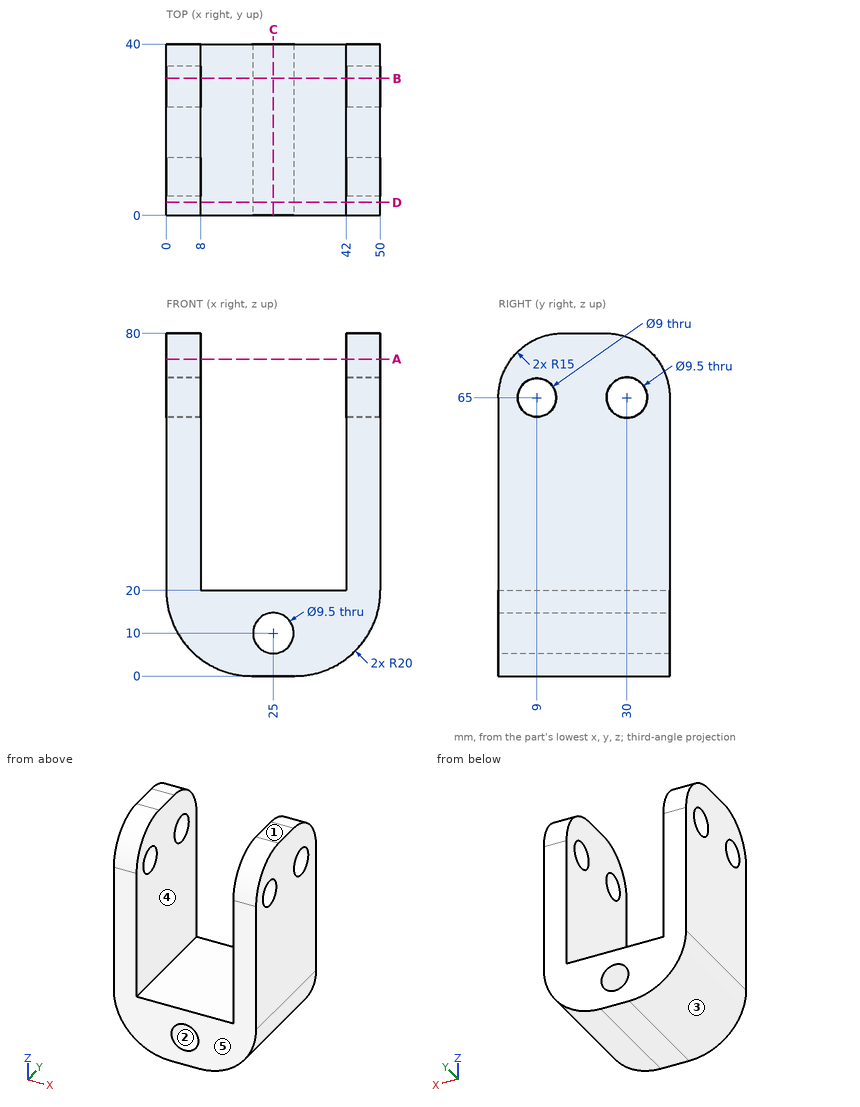
Geometry: see drawing. Coordinates: mm, zero at the bounding-box minimum. A direction names the side the tool comes from. Round coordinates to 2 decimals unless told otherwise and drop trailing zeros. Loops run counter-clockwise (first coordinate to the right, second up) from the corner with the lowest first, then second, coordinate; pieces in that order, holes last. Notation, with made-up numbers: M 4.5,52.25 L 54.5,52.25 A28 cw 54.5,85.25 Z; hole C 45,-9 d4. An arc over 180 degrees is marked long. Use a Markdown table: item, result. Add a question column.
1. Contact query for flat-ended pins moving along their axis: P1, Ø8.5, axis at y = 30, z = 65, coming from the -X side; P2, Ø10, axis at x = 24, y = 31, coming from the +Z side; P3, Ø10, axis at x = 44, y = 35, coming from the +Z side; P4, Ø10, axis at x = 11, y = 4.5, coming from the -Z side. Output: stop coordinate, or through.
2. Section query D-D on y = 3. Return the cut outline in (x, z), then the cut area to 3 significant figures.
3. Section query B-B on y = 32. Return the cut outline in (x, z).
4. Section query A-A on z = 74. Return the cut outline in (x, y).
5. Line query: line 1 (Y direction, x = 3.75, z = 65); line 2 (X direction, y = 25, z = 45); line 3 (Z direction, x = 42.5, y = 32). Output: solid intervals per line, ascending.
6. Reachability of the marked faces 4 and 5 from +Z, -Z, +X, -X, +Y, -Y: full face, straight path, thin tool, end or side. Return the list, or none.
7. Mould query, pull axis X, two halves, no side actions, for the marked faces 1, 2 and 3. Classes: pulls with the +X half, pulls with the -X half, needs draft (parallel to the pull), parting line crosses it, or undercut.
8. Section query C-C on x = 25. Return the cut outline in (y, z).
Reported:
| question | item | result |
|---|---|---|
| 1 | P1 | passes through |
| 1 | P2 | stops at z = 20 |
| 1 | P3 | stops at z = 79.14 |
| 1 | P4 | stops at z = 0.4 |
| 2 | outline | M 0,20 A20 ccw 20,0 L 30,0 A20 ccw 50,20 L 50,74 L 42,74 L 42,20 L 8,20 L 8,74 L 0,74 Z; hole C 25,10 d9.5 |
| 2 | area | 1,620 mm² |
| 3 | outline | M 0,20 A20 ccw 20,0 L 30,0 A20 ccw 50,20 L 50,60.69 L 42,60.69 L 42,20 L 8,20 L 8,60.69 L 0,60.69 Z; M 0,69.31 L 8,69.31 L 8,78.27 L 0,78.27 Z; M 42,69.31 L 50,69.31 L 50,78.27 L 42,78.27 Z; hole C 25,10 d9.5 |
| 4 | outline | M 0,3 L 8,3 L 8,37 L 0,37 Z; M 42,3 L 50,3 L 50,37 L 42,37 Z |
| 5 | line 1 | y = 0 to 4.5, 13.5 to 25.25, 34.75 to 40 |
| 5 | line 2 | x = 0 to 8, 42 to 50 |
| 5 | line 3 | z = 4.39 to 60.69, 69.31 to 78.27 |
| 6 | face 4 | +Z, +Y, -Y |
| 6 | face 5 | +Z, -Z, +X, -X, -Y |
| 7 | face 1 | needs draft |
| 7 | face 2 | undercut |
| 7 | face 3 | pulls with the -X half |
| 8 | outline | M 0,0 L 40,0 L 40,5.25 L 0,5.25 Z; M 0,14.75 L 40,14.75 L 40,20 L 0,20 Z |
